Check sheet for the modelled part. Datum: model origin and axes. Units: mm. Coordinates: 2 decimals unless noted, no trailing zeros. Loops run counter-clockwise (first coordinate to the right, second up) from the corner with the lowest first, then second, coordinate; pieces in that order, holes last.
```python
from build123d import *

# Parameters (mm, degrees)
SKETCH1_W           = 150
SKETCH1_H           = 270
BOSS_EXTRUDE1_DEPTH = 6.35
SKETCH2_R           = 2.25
SKETCH2_R_2         = 30
CUT_EXTRUDE1_DEPTH  = 7.35
SKETCH6_R           = 0.85
CUT_EXTRUDE5_DEPTH  = 7.35
SKETCH7_R           = 1.7
CUT_EXTRUDE6_DEPTH  = 7.35
SKETCH8_R           = 25
CUT_EXTRUDE9_DEPTH  = 7.35


with BuildPart() as part:
    # Sketch1 → Boss-Extrude1 (new body)
    with BuildSketch(Plane(origin=(0, 0, 0), x_dir=(1, 0, 0), z_dir=(0, 1, 0))):
        Rectangle(SKETCH1_W, SKETCH1_H)
    extrude(amount=BOSS_EXTRUDE1_DEPTH)

    # Sketch2 → Cut-Extrude1 (cut, through all)
    with BuildSketch(Plane(origin=(0, 6.35, 0), x_dir=(1, 0, 0), z_dir=(0, 1, 0))):
        with Locations((0, -18.5)):
            Circle(SKETCH2_R)
        with Locations((29.344931419, -30.655068581)):
            Circle(SKETCH2_R)
        with Locations((41.5, -60)):
            Circle(SKETCH2_R)
        with Locations((29.344931419, -89.344931419)):
            Circle(SKETCH2_R)
        with Locations((0, -101.5)):
            Circle(SKETCH2_R)
        with Locations((-29.344931419, -89.344931419)):
            Circle(SKETCH2_R)
        with Locations((-41.5, -60)):
            Circle(SKETCH2_R)
        with Locations((-29.344931419, -30.655068581)):
            Circle(SKETCH2_R)
        with Locations((0, -60)):
            Circle(SKETCH2_R_2)
    extrude(amount=-CUT_EXTRUDE1_DEPTH, mode=Mode.SUBTRACT)

    # Sketch6 → Cut-Extrude5 (cut, through all)
    with BuildSketch(Plane(origin=(0, 6.35, 0), x_dir=(1, 0, 0), z_dir=(0, 1, 0))):
        with Locations((-36.963798099, -37.522452757)):
            Circle(SKETCH6_R)
        with Locations((-40.978671586, -46.132376734)):
            Circle(SKETCH6_R)
        with Locations((-29.908156972, -46.053597363)):
            Circle(SKETCH6_R)
    extrude(amount=-CUT_EXTRUDE5_DEPTH, mode=Mode.SUBTRACT)

    # Sketch7 → Cut-Extrude6 (cut, through all)
    with BuildSketch(Plane(origin=(0, 6.35, 0), x_dir=(1, 0, 0), z_dir=(0, 1, 0))):
        with Locations((-64.5, -127.5)):
            Circle(SKETCH7_R)
        with Locations((-21.5, -127.5)):
            Circle(SKETCH7_R)
        with Locations((21.5, -127.5)):
            Circle(SKETCH7_R)
        with Locations((64.5, -127.5)):
            Circle(SKETCH7_R)
        with Locations((64.5, 127.5)):
            Circle(SKETCH7_R)
        with Locations((21.5, 127.5)):
            Circle(SKETCH7_R)
        with Locations((-64.5, 127.5)):
            Circle(SKETCH7_R)
        with Locations((-21.5, 127.5)):
            Circle(SKETCH7_R)
    extrude(amount=-CUT_EXTRUDE6_DEPTH, mode=Mode.SUBTRACT)

    # Sketch8 → Cut-Extrude9 (cut, through all)
    with BuildSketch(Plane(origin=(0, 6.35, 0), x_dir=(1, 0, 0), z_dir=(0, 1, 0))):
        with Locations((0, 70)):
            Circle(SKETCH8_R)
    extrude(amount=-CUT_EXTRUDE9_DEPTH, mode=Mode.SUBTRACT)


solid = part.part
```
1) Section check D-D on z = 82.5. Enter the section's corners in (x, y), plus the area to 3 significant figures.
Answer sheet:
outline: (-75, 0) - (-19.84, 0) - (-19.84, 6.35) - (-75, 6.35) - close; (19.84, 0) - (75, 0) - (75, 6.35) - (19.84, 6.35) - close
area: 700 mm2
2) Section check C-C on y = 2.5. Give the number of separate pieces and of enclosed holes in the cut face, plus the area to 3 significant figures.
Answer sheet:
separate pieces: 1
enclosed holes: 21
area: 35,500 mm2
3) Section check A-A on z = -70. Enter the section's corners in (x, y), plus the area to 3 significant figures.
Answer sheet:
outline: (-75, 0) - (-25, 0) - (-25, 6.35) - (-75, 6.35) - close; (25, 0) - (75, 0) - (75, 6.35) - (25, 6.35) - close
area: 635 mm2
4) Section check B-B on x = -14.5. Enter the section's corners in (y, z).
Answer sheet:
outline: (0, -135) - (6.35, -135) - (6.35, -90.37) - (0, -90.37) - close; (0, -49.63) - (6.35, -49.63) - (6.35, 33.74) - (0, 33.74) - close; (0, 86.26) - (6.35, 86.26) - (6.35, 135) - (0, 135) - close
5) Depth check by flat-ended pin: pin 1 (4 mm diameter, centred on x = -29.34, z = 30.66, fed in from +Y). Enter the tip coordinate at first touch or a pass-through.
Answer sheet:
pin 1: passes through
6) Mould release check, pull along X, two halves, no side actions. Record for faces 1 (the cylindrical face through (-5.42, 3.219, -45.594)), 2 (the cylindrical face through (-6.503, 3.219, 89.287)), 3 (the flat face through (-75, 3, 2)), 4 (the flat face through (75, 3, 2)): +X half, -X half, draft (parallel to the pull), parting line (faces both ways), or undercut.
Answer sheet:
face 1: undercut
face 2: undercut
face 3: -X half
face 4: +X half
7) Scan lines: line 1 (X direction, y = 1.5, z = -127.5); line 2 (X direction, y = 3.5, z = 60); line 3 (Z direction, x = 64.5, y = 2). Record each from-to range of solid material in increasing order.
Answer sheet:
line 1: x = -75 to -66.2, -62.8 to -23.2, -19.8 to 19.8, 23.2 to 62.8, 66.2 to 75
line 2: x = -75 to -43.75, -39.25 to -30, 30 to 39.25, 43.75 to 75
line 3: z = -135 to -129.2, -125.8 to 125.8, 129.2 to 135
